Verification items for the finished model (mm, model axes). A direction names the side the tool comes from. Coordinates: 2 decimals unless noted, no trailing zeros. Loops run counter-clockwise (first coordinate to the right, second up) from the corner with the lowest first, then second, coordinate; pieces in that order, holes last. Notation, with made-up numbers: (-40, 52.5) - (-5, 52.5) arc R11 cw to (-5, 68.5) - close; hole circle Ø6 at (7, -39). An arc over 180 degrees is marked (long way). Answer as CSV lines item,"result". Start each with the question number.
1. Gauge pin test, flat ends, axial feed: P1, Ø1.5, axis at x = -23.5, y = 36.5, coming from the +Z side; P2, Ø10, axis at x = 1.5, z = 57.5, coming from the +Y side; P3, Ø1, axis at y = 21.5, z = 9.5, coming from the -X side. Record the tip position at first contact, or that the pin passes through.
2. Cross-section at A-A (y = -42). Enter the section's corners in (x, z).
3. Cross-section at B-B (x = -39). Enter the section's corners in (y, z).
4. Material ranges on line 1 (Y direction, x = 0, z = -1); line 2 (Z direction, x = -33.5, y = 9.5); line 3 (Y direction, x = 16.5, z = 25), recorded low to high. Write a range as [from, to].
5. Cross-section at D-D (z = 15). Enter the section's corners in (x, y).
6. Cross-section at C-C (y = 0). Enter the section's corners in (x, z), plus the area to 3 significant figures.
7. Set-up check for faces 1 (the cylindrical face through (22.013, 33.338, -1.282)), 2 (the flat face through (23, -23, 0)): record each of +Z, -Z, +X, -X, +Y, -Y from which the full face is reachable in a straight line by a thin tool's end or side.
8. Release check for a two-part mould opening along X. For faces 3 (the flat face through (-1, 1, -2.6)), 4 (the cylindrical face through (-37.404, -14.032, -1.282)), 5 (the cylindrical face through (-5.85, -26.36, 39.44)) record: pulls with the +X half, pulls with the -X half, needs draft (parallel to the pull), parting line crosses it, or undercut.
```python
from build123d import *

# Parameters (mm, degrees)
SKETCH1_R           = 52.5
BOSS_EXTRUDE1_DEPTH = 2.6
SKETCH2_R           = 27
BOSS_EXTRUDE2_DEPTH = 80
SKETCH3_R           = 2.75
CUT_EXTRUDE1_DEPTH  = 110.144399765
CIRPATTERN1_COUNT   = 5


with BuildPart() as part:
    # Sketch1 → Boss-Extrude1 (new body)
    with BuildSketch(Plane.XY):
        Circle(SKETCH1_R)
    extrude(amount=-BOSS_EXTRUDE1_DEPTH)

    # Sketch2 → Boss-Extrude2 (add)
    with BuildSketch(Plane.XY):
        Circle(SKETCH2_R)
    extrude(amount=BOSS_EXTRUDE2_DEPTH)

    # Sketch3 → Cut-Extrude1 (cut, through all)
    with BuildSketch(Plane.XY):
        with Locations((-39.944373684, -12.978713764)):
            Circle(SKETCH3_R)
    cut_extrude1 = extrude(amount=-CUT_EXTRUDE1_DEPTH, mode=Mode.SUBTRACT)

    # CirPattern1: Cut-Extrude1 ×5 about axis
    cirpattern1_axis = Axis((0, 0, 0), (0, 0, 1))
    for i in range(1, CIRPATTERN1_COUNT):
        add(cut_extrude1.rotate(cirpattern1_axis, i * 360 / CIRPATTERN1_COUNT), mode=Mode.SUBTRACT)


solid = part.part
```
Values follow:
1,P1,"stops at z = 0"
1,P2,"stops at y = 27"
1,P3,"stops at x = -16.97"
2,outline,"(-31.5, -2.6) - (-2.75, -2.6) - (-2.75, 0) - (-31.5, 0) - close; (2.75, -2.6) - (31.5, -2.6) - (31.5, 0) - (2.75, 0) - close"
3,outline,"(-35.15, -2.6) - (-15.56, -2.6) - (-15.56, 0) - (-35.15, 0) - close; (-10.4, -2.6) - (35.15, -2.6) - (35.15, 0) - (-10.4, 0) - close"
4,line 1,"y = [-52.5, -44.75], [-39.25, 52.5]"
4,line 2,"z = [-2.6, 0]"
4,line 3,"y = [-21.37, 21.37]"
5,outline,"circle Ø54 at (0, 0)"
6,outline,"(-52.5, -2.6) - (52.5, -2.6) - (52.5, 0) - (27, 0) - (27, 80) - (-27, 80) - (-27, 0) - (-52.5, 0) - close"
6,area,"4,590 mm²"
7,face 1,"+Z, -Z"
7,face 2,"+Z"
8,face 3,"needs draft"
8,face 4,"undercut"
8,face 5,"parting line crosses it"
